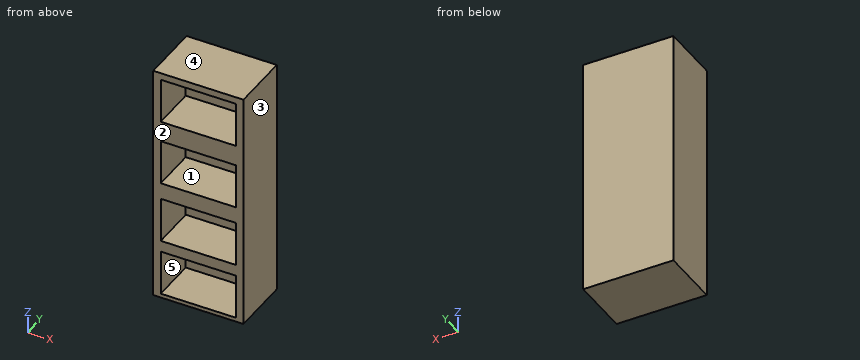
```python
from build123d import *

# Parameters (mm, degrees)
F0_W     = 457.2
F0_H     = 304.8
F1_DEPTH = 1219.2
F2_W     = 381
F2_H     = 228.6
F3_DEPTH = 228.6


with BuildPart() as f1:
    # F0 (on Top) → F1 (new body)
    with BuildSketch(Plane.XY):
        with Locations((-25.902518, 25.154568)):
            Rectangle(F0_W, F0_H)
    extrude(amount=F1_DEPTH)

    # F2 (on face) → F3 (cut)
    with BuildSketch(Plane.XZ.offset(127.245432)):
        with Locations((-25.902518, 1069.40844)):
            Rectangle(F2_W, F2_H)
        with Locations((-25.902518, 735.381065)):
            Rectangle(F2_W, F2_H)
        with Locations((-25.902518, 422.230378)):
            Rectangle(F2_W, F2_H)
        with Locations((-25.902518, 135.175608)):
            Rectangle(F2_W, F2_H)
    extrude(amount=-F3_DEPTH, mode=Mode.SUBTRACT)


solid = f1.part
```
Check sheet for the modelled part. Datum: model origin and axes. Units: mm. Face numbers are marked on the shaded views. A direction names the side the tool comes from. Give positions to 0.01 mm unless a question says otherwise; leave off trailing zeros. Order: outer loops, then holes, each group sorted by start corner. A loop starts at its lowest first (then second) coordinate and runs counter-clockwise, first axis right, second up. Notation, with made-up numbers: M 84.5,43.5 L 96.5,43.5 A13 cw 96.5,54.5 Z; hole C -23.75,48 d7. An arc over 180 degrees is marked long. Answer in a Markdown table with one row per item. Add a question column.
Q1. Release check for a two-part mould opening along X. For the marked faces 1, 2 and 3 record: released by +X, released by -X, zero draft, split by the parting line, or undercut.
Q2. Sectioned sample at C-C, the plane x = -138. Record the boundary of the cut face in (y, z).
Q3. Gauge pin test, flat ends, axial feed: pin 1 Ø3 at (x, y) = (-103, -46) entering from -Z; pin 2 Ø10 at (x, z) = (65, 704.5) entering from -Y. Record the tip position at first contact, or that the pin passes through.
Q4. Access from +Z, -Z, +X, -X, +Y, -Y to the whole of each face (thin tool, end or side, straight path). Record for the marked faces 4 and 5.
Q5. Thickness scan on L1, parallel to Z at x = -139, y = 33.5; L2, parallel to X at y = -59, z = 718.5; L3, parallel to Y at x = -104, z = 987. Record the ranges inside material, lowest first.
Q6. Sectioned sample at B-B, the plane z = 814. Record the boundary of the cut face in (x, y), and give its area (3 significant figures).
Q7. Sectioned sample at A-A, the plane y = -9. Record the boundary of the cut face in (x, z), and give its area (3 significant figures).
Verdict:
| question | item | result |
|---|---|---|
| 1 | face 1 | undercut |
| 1 | face 2 | zero draft |
| 1 | face 3 | released by +X |
| 2 | outline | M -127.25,0 L 177.55,0 L 177.55,1219.2 L -127.25,1219.2 L -127.25,1183.71 L 101.35,1183.71 L 101.35,955.11 L -127.25,955.11 L -127.25,849.68 L 101.35,849.68 L 101.35,621.08 L -127.25,621.08 L -127.25,536.53 L 101.35,536.53 L 101.35,307.93 L -127.25,307.93 L -127.25,249.48 L 101.35,249.48 L 101.35,20.88 L -127.25,20.88 Z |
| 3 | pin 1 | z = 0 |
| 3 | pin 2 | y = 101.35 |
| 4 | face 4 | +Z, +X, -X, +Y, -Y |
| 4 | face 5 | -Y |
| 5 | L1 | 0 to 20.88, 249.48 to 307.93, 536.53 to 621.08, 849.68 to 955.11, 1183.71 to 1219.2 |
| 5 | L2 | -254.5 to -216.4, 164.6 to 202.7 |
| 5 | L3 | 101.35 to 177.55 |
| 6 | outline | M -254.5,-127.25 L -216.4,-127.25 L -216.4,101.35 L 164.6,101.35 L 164.6,-127.25 L 202.7,-127.25 L 202.7,177.55 L -254.5,177.55 Z |
| 6 | area | 52,300 mm² |
| 7 | outline | M -254.5,0 L 202.7,0 L 202.7,1219.2 L -254.5,1219.2 Z; hole M -216.4,20.88 L 164.6,20.88 L 164.6,249.48 L -216.4,249.48 Z; hole M -216.4,307.93 L 164.6,307.93 L 164.6,536.53 L -216.4,536.53 Z; hole M -216.4,621.08 L 164.6,621.08 L 164.6,849.68 L -216.4,849.68 Z; hole M -216.4,955.11 L 164.6,955.11 L 164.6,1183.71 L -216.4,1183.71 Z |
| 7 | area | 209,000 mm² |
